Read the model definition and answer for the solid it produces. Units are mm, in the model's axes. Give positions to 0.01 mm unless a question says otherwise; leave off trailing zeros. Loops run counter-clockwise (first coordinate to the right, second up) from the corner with the lowest first, then second, coordinate; pieces in that order, holes last. Notation, with made-up numbers: (-16, -32.5) - (30, -32.5) arc R31 cw to (30, -1.5) - close; hole circle Ø5 at (15.25, 65). An arc over 180 degrees is marked (long way). Put each result on its own line as item: value. Start each with the question number.
1. A cutting plane is placed at D-D, the plane x = 2. Determine the outline of the cut face in (y, z), plus the area to 3 significant figures.
2. Consider L1, parallel to Y at x = -5.75, z = 0.5; L2, parallel to X at y = -1.3, z = -6; L3, parallel to X at y = 10.75, z = -7.25. Determine where each line is inside the solid, lowest interval first. Write a range as from..to.
3. Given pin 1 Ø2.5 at (y, z) = (6, -4.5) entering from -X, flat-ended and moving along its own axis, determine where the tip first touches the part or whether it passes through.
4. For a pull along Y with two mould halves and no side action, classify faces 1 (the cylindrical face through (0, 5, 4)), 2 (the flat face through (8, -1, -2)), 3 (the flat face through (0, -2, -1)) as released by +Y, released by -Y, zero draft, split by the parting line, or undercut.
5. A cutting plane is placed at A-A, the plane y = -0.75. Determine the outline of the cut face in (x, z).
6. A cutting plane is placed at B-B, the plane z = 0. Determine the outline of the cut face in (x, y).
7. A cutting plane is placed at C-C, the plane x = 6.5. Determine the outline of the cut face in (y, z), plus the area to 3 significant figures.
```python
from build123d import *
from build123d.topology import SkipClean

# Parameters (mm, degrees)
BOSS_EXTRUDE1_DEPTH = 10
BOSS_EXTRUDE2_DEPTH = 2
FILLET1_R           = 3.2
BOSS_EXTRUDE4_START = 2
BOSS_EXTRUDE4_DEPTH = 2
FILLET3_R           = 2
SKETCH5_R           = 1.5
CUT_EXTRUDE1_DEPTH  = 14


with BuildPart() as part:
    # Sketch1 → Boss-Extrude1 (new body)
    with BuildSketch(Plane(origin=(0, 0, 0), x_dir=(1, 0, 0), z_dir=(0, 1, 0))):
        with BuildLine():
            Line((-3.2, 7.4), (-3.2, 4))
            Line((-3.2, 4), (-3.2, -4))
            Line((-3.2, -4), (3.2, -4))
            Line((3.2, -4), (3.2, 4))
            Line((3.2, 4), (3.2, 7.4))
            ThreePointArc((3.2, 7.4), (0, 4.2), (-3.2, 7.4))
        make_face()
    extrude(amount=BOSS_EXTRUDE1_DEPTH)

    # Sketch2 → Boss-Extrude2 (add)
    with SkipClean():  # the faces are left unmerged after this step: merging them gives an invalid solid
        with BuildSketch(Plane(origin=(0, 10, 0), x_dir=(1, 0, 0), z_dir=(0, 1, 0))):
            with BuildLine():
                Line((-8, 8), (-3.143246729, 8))
                ThreePointArc((-3.143246729, 8), (0, 4.2), (3.143246729, 8))
                Line((3.143246729, 8), (8, 8))
                Line((8, 8), (8, -4))
                Line((8, -4), (-8, -4))
                Line((-8, -4), (-8, 8))
            make_face()
        extrude(amount=BOSS_EXTRUDE2_DEPTH)

    # Fillet1
    # the kernel refuses this fillet: 3.2 mm, written as the material it takes off along each edge
    with BuildSketch(Plane(origin=(-3.2, -8, 4), x_dir=(0, 0, -1), z_dir=(0, 1, 0)), Plane(origin=(3.2, -8, 4), x_dir=(-1, 0, 0), z_dir=(0, 1, 0))) as fillet1_piece_1:
        with BuildLine():
            CenterArc((FILLET1_R, -FILLET1_R), FILLET1_R, 90, 90)
            Line((0, -FILLET1_R), (0, 0))
            Line((0, 0), (FILLET1_R, 0))
        make_face()
    extrude(amount=18, mode=Mode.SUBTRACT)

    # Sketch3 → Boss-Extrude4 (add)
    with SkipClean():  # the faces are left unmerged after this step: merging them gives an invalid solid
        with BuildSketch(Plane.XZ.offset(BOSS_EXTRUDE4_START)):
            with BuildLine():
                Line((8, 4), (-8, 4))
                Line((-8, 4), (-8, -8))
                Line((-8, -8), (-3.143246729, -8))
                ThreePointArc((-3.143246729, -8), (0, -4.2), (3.143246729, -8))
                Line((3.143246729, -8), (8, -8))
                Line((8, -8), (8, 4))
            make_face()
        extrude(amount=-BOSS_EXTRUDE4_DEPTH)

    # Fillet3
    fillet3_edges = [part.edges().sort_by_distance(p)[0] for p in [
        (-8, 11, -8),
        (-8, 11, 4),
        (8, 11, 4),
        (8, 11, -8),
        (8, -1, -8),
        (8, -1, 4),
        (-8, -1, 4),
        (-8, -1, -8),
    ]]
    fillet(fillet3_edges, radius=FILLET3_R)

    # Sketch5 → Cut-Extrude1 (cut)
    with SkipClean():  # the faces are left unmerged after this step: merging them gives an invalid solid
        with BuildSketch(Plane(origin=(0, 12, 0), x_dir=(1, 0, 0), z_dir=(0, 1, 0))):
            with Locations(Location((-6, 6, 0), (0, 0, 270))):
                Circle(SKETCH5_R)
            with Locations(Location((6, 6, 0), (0, 0, 270))):
                Circle(SKETCH5_R)
        extrude(amount=-CUT_EXTRUDE1_DEPTH, mode=Mode.SUBTRACT)


solid = part.part
```
Return value:
1. outline: (-2, -4.9) - (12, -4.9) - (12, 4) - (10, 4) - (10, 3.3) - (0, 3.3) - (0, 4) - (-2, 4) - close
1. area: 118 mm2
2. L1: y = -2..0, 10..12
2. L2: x = -8..-7.5, -4.5..-2.88, 2.88..4.5, 7.5..8
2. L3: x = -7.56..-6.83, -5.17..-3.2, 3.2..5.17, 6.83..7.56
3. pin 1: stops at x = -3.2
4. face 1: undercut
4. face 2: zero draft
4. face 3: released by -Y
5. outline: (-8, -6) arc R2 ccw to (-6, -8) - (-3.14, -8) arc R3.2 cw (long way) to (3.14, -8) - (6, -8) arc R2 ccw to (8, -6) - (8, 2) arc R2 ccw to (6, 4) - (-6, 4) arc R2 ccw to (-8, 2) - close; hole circle Ø3 at (-6, -6); hole circle Ø3 at (6, -6)
6. outline: (-8, -2) - (8, -2) - (8, 0) - (3.2, 0) - (3.2, 10) - (8, 10) - (8, 12) - (-8, 12) - (-8, 10) - (-3.2, 10) - (-3.2, 0) - (-8, 0) - close
7. outline: (-2, -7.94) - (0, -7.94) - (0, -7.41) - (-2, -7.41) - close; (-2, -4.59) - (0, -4.59) - (0, 3.94) - (-2, 3.94) - close; (10, -7.94) - (12, -7.94) - (12, -7.41) - (10, -7.41) - close; (10, -4.59) - (12, -4.59) - (12, 3.94) - (10, 3.94) - close
7. area: 36.2 mm2
